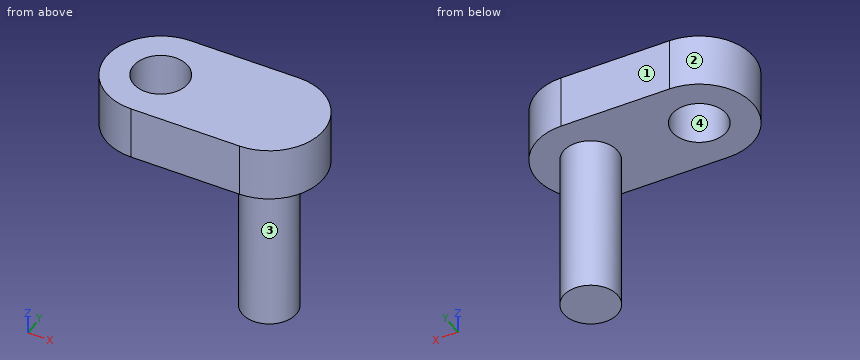
from build123d import *

# Parameters (mm, degrees)
SKETCH1_R           = 2.5
BOSS_EXTRUDE1_DEPTH = 5
SKETCH1_3_R         = 2.5
BOSS_EXTRUDE2_DEPTH = 15


with BuildPart() as part:
    # Sketch1 → Boss-Extrude1 (new body)
    with BuildSketch(Plane.XY):
        with BuildLine():
            Line((-13.904710079, 5), (-3.904710079, 5))
            ThreePointArc((-3.904710079, 5), (1.095289921, 0), (-3.904710079, -5))
            Line((-3.904710079, -5), (-13.904710079, -5))
            ThreePointArc((-13.904710079, -5), (-18.904710079, 0), (-13.904710079, 5))
        make_face()
        with Locations((-13.904710079, 0)):
            Circle(SKETCH1_R, mode=Mode.SUBTRACT)
    extrude(amount=BOSS_EXTRUDE1_DEPTH)

    # Sketch1<3> → Boss-Extrude2 (add)
    with BuildSketch(Plane.XY):
        with Locations((-3.904710079, 0)):
            Circle(SKETCH1_3_R)
    extrude(amount=-BOSS_EXTRUDE2_DEPTH)


solid = part.part
Here's how the part is built. I have some questions about the finished solid (model axes, mm). Face numbers are marked on the shaded views. Round coordinates to 2 decimals unless told otherwise and drop trailing zeros. Loops run counter-clockwise (first coordinate to the right, second up) from the corner with the lowest first, then second, coordinate; pieces in that order, holes last. Notation, with made-up numbers: (34, -36.75) - (41, -36.75) arc R22 ccw to (41, -4.75) - close; hole circle Ø7 at (71.5, 65.5). An arc over 180 degrees is marked (long way). One line per question, with ' | ' between items. Start each with the question number.
Q1. I want a section at B-B (y = 1.5). Write out the boundary of the cut face in (x, z), then the cut area to 3 significant figures.
Q2. We'd pull the mould along X, two halves only. Please class the marked faces 1, 2, 3 and 4: +X half, -X half, draft (parallel to the pull), parting line (faces both ways), or undercut.
Q3. Please list where these lines run through material, in increasing order: line 1 (Z direction, x = -0.5, y = 1.25); line 2 (X direction, y = 2, z = 0.75); line 3 (Y direction, x = -4, z = -1.5). Write a range as [from, to].
Q4. I want a section at A-A (y = 0). Write out the boundary of the cut face in (x, z), then the cut area to 3 significant figures.
Q5. Will these pins go through, and if not, where does the flat tip stop? pin 1 (6 mm diameter, centred on x = -9, z = -2.5, fed in from -Y); pin 2 (1.5 mm diameter, centred on y = -3.5, z = -8.5, fed in from +X); pin 3 (2 mm diameter, centred on y = 1, z = -6.5, fed in from -X).
Q6. I want a section at D-D (x = -9.75). Write out the boundary of the cut face in (y, z), then the cut area to 3 significant figures.
Q7. I want a section at C-C (z = -10). Write out the boundary of the cut face in (x, y).
Response values:
1) outline: (-18.67, 0) - (-15.9, 0) - (-15.9, 5) - (-18.67, 5) - close; (-11.9, 0) - (-5.9, 0) - (-5.9, -15) - (-1.9, -15) - (-1.9, 0) - (0.86, 0) - (0.86, 5) - (-11.9, 5) - close | area: 138 mm²
2) face 1: draft | face 2: -X half | face 3: parting line | face 4: undercut
3) line 1: z = [0, 5] | line 2: x = [-18.49, -15.4], [-12.4, 0.68] | line 3: y = [-2.5, 2.5]
4) outline: (-18.9, 0) - (-16.4, 0) - (-16.4, 5) - (-18.9, 5) - close; (-11.4, 0) - (-6.4, 0) - (-6.4, -15) - (-1.4, -15) - (-1.4, 0) - (1.1, 0) - (1.1, 5) - (-11.4, 5) - close | area: 150 mm²
5) pin 1: stops at y = -5 | pin 2: passes through | pin 3: stops at x = -6.4
6) outline: (-5, 0) - (5, 0) - (5, 5) - (-5, 5) - close | area: 50.0 mm²
7) outline: circle Ø5 at (-3.9, 0)
